from build123d import *

# Parameters (mm, degrees)
SKETCH_1_W          = 55
SKETCH_1_H          = 85
EXTRUDE_1_DEPTH     = 5
SKETCH_2_W          = 7
SKETCH_2_H          = 6.5
EXTRUDE_2_DEPTH     = 26
SKETCH_3_R          = 1.475
CUT_EXTRUDE_1_DEPTH = 103.30377559
SKETCH_4_W          = 41
SKETCH_4_H          = 15
EXTRUDE_3_DEPTH     = 7.75
SKETCH_5_W          = 24.5
SKETCH_5_H          = 49.5
EXTRUDE_4_DEPTH     = 10
SKETCH_7_R          = 2.525
CUT_EXTRUDE_2_DEPTH = 2.25
SKETCH_8_W          = 2.7
SKETCH_8_H          = 15.4
CUT_EXTRUDE_3_DEPTH = 12
SKETCH_9_W          = 1.9
SKETCH_9_H          = 14.5
CUT_EXTRUDE_4_DEPTH = 1
SKETCH_10_W         = 10
SKETCH_10_H         = 14.5
CUT_EXTRUDE_5_DEPTH = 70.787624261
FILLET_1_R          = 3
FILLET_2_R          = 7.5


with BuildPart() as part:
    # Эскиз1 → Бобышка-Вытянуть1 (new body)
    with BuildSketch(Plane(origin=(0, 0, 0), x_dir=(1, 0, 0), z_dir=(0, 1, 0))):
        with Locations((-20.25, 0)):
            Rectangle(SKETCH_1_W, SKETCH_1_H)
    extrude(amount=EXTRUDE_1_DEPTH)

    # Эскиз2 → Бобышка-Вытянуть2 (add)
    with BuildSketch(Plane(origin=(0, 5, 0), x_dir=(1, 0, 0), z_dir=(0, 1, 0))):
        with Locations((-44.25, 39.25)):
            Rectangle(SKETCH_2_W, SKETCH_2_H)
        with Locations((3.75, 39.25)):
            Rectangle(SKETCH_2_W, SKETCH_2_H)
        with Locations((3.75, -39.25)):
            Rectangle(SKETCH_2_W, SKETCH_2_H)
        with Locations((-44.25, -39.25)):
            Rectangle(SKETCH_2_W, SKETCH_2_H)
    extrude(amount=EXTRUDE_2_DEPTH)

    # Эскиз3 → Вырез-Вытянуть1 (cut, through all)
    with BuildSketch(Plane.XY.offset(42.5)):
        with Locations((-44.55, 28)):
            Circle(SKETCH_3_R)
        with Locations((-44.55, 18)):
            Circle(SKETCH_3_R)
        with Locations((4.05, 18)):
            Circle(SKETCH_3_R)
        with Locations((4.05, 28)):
            Circle(SKETCH_3_R)
    extrude(amount=-CUT_EXTRUDE_1_DEPTH, mode=Mode.SUBTRACT)

    # Эскиз4 → Бобышка-Вытянуть3 (add)
    with BuildSketch(Plane(origin=(0, 5, 0), x_dir=(1, 0, 0), z_dir=(0, 1, 0))):
        with Locations((-20.25, 35)):
            Rectangle(SKETCH_4_W, SKETCH_4_H)
        with Locations((-20.25, -35)):
            Rectangle(SKETCH_4_W, SKETCH_4_H)
    extrude(amount=EXTRUDE_3_DEPTH)

    # Эскиз5 → Бобышка-Вытянуть4 (add)
    with BuildSketch(Plane.XZ):
        with Locations((-20.25, 0)):
            Rectangle(SKETCH_5_W, SKETCH_5_H)
    extrude(amount=EXTRUDE_4_DEPTH)

    # Эскиз7 → Вырез-Вытянуть2 (cut)
    with BuildSketch(Plane.XZ.offset(10)):
        with Locations(Location((-13, 20, 0), (0, 0, 270))):
            Circle(SKETCH_7_R)
        with Locations(Location((-13, -20, 0), (0, 0, 270))):
            Circle(SKETCH_7_R)
    extrude(amount=-CUT_EXTRUDE_2_DEPTH, mode=Mode.SUBTRACT)

    # Эскиз8 → Вырез-Вытянуть3 (cut)
    with BuildSketch(Plane.XZ.offset(10)):
        with Locations((-29, 0)):
            Rectangle(SKETCH_8_W, SKETCH_8_H)
        with Locations((-25, 0)):
            Rectangle(SKETCH_8_W, SKETCH_8_H)
    extrude(amount=-CUT_EXTRUDE_3_DEPTH, mode=Mode.SUBTRACT)

    # Эскиз9 → Вырез-Вытянуть4 (cut)
    with BuildSketch(Plane.XZ.offset(-2)):
        with Locations((-29, 0)):
            Rectangle(SKETCH_9_W, SKETCH_9_H)
        with Locations((-25, 0)):
            Rectangle(SKETCH_9_W, SKETCH_9_H)
    extrude(amount=-CUT_EXTRUDE_4_DEPTH, mode=Mode.SUBTRACT)

    # Эскиз10 → Вырез-Вытянуть5 (cut, through all)
    with BuildSketch(Plane.XZ.offset(-3)):
        with Locations((-24.95, 0)):
            Rectangle(SKETCH_10_W, SKETCH_10_H)
    extrude(amount=-CUT_EXTRUDE_5_DEPTH, mode=Mode.SUBTRACT)

    # Скругление1
    fillet_1_edges = [part.edges().sort_by_distance(p)[0] for p in [
        (-32.5, -5, 24.75),
        (-32.5, -5, -24.75),
        (-8, -5, -24.75),
        (-8, -5, 24.75),
    ]]
    fillet(fillet_1_edges, radius=FILLET_1_R)

    # Скругление2
    fillet_2_edges = [part.edges().sort_by_distance(p)[0] for p in [
        (-20.25, 5, -27.5),
        (-20.25, 5, 27.5),
        (-44.25, 5, 36),
        (3.75, 5, 36),
        (3.75, 5, -36),
        (-44.25, 5, -36),
    ]]
    fillet(fillet_2_edges, radius=FILLET_2_R)


solid = part.part
Model file for the job. Use its own axes, mm. A direction names the side the tool comes from. Give positions to 0.01 mm unless a question says otherwise; leave off trailing zeros. Write each loop counter-clockwise with the first axis right and the second up, starting at its lowest first coordinate (ties: lowest second). Pieces come first, ordered by that corner, then holes. Notation, with made-up numbers: M 12,-8.5 L 16,-8.5 A20 ccw 16,12.5 Z; hole C 10,71 d10. An arc over 180 degrees is marked long. One line per item, written item: value. Start each with the question number.
Q1. Saw through at C-C, the plane z = 0. Write the cut outline in (x, y), plus the area to 3 significant figures.
Q2. Saw through at B-B, the plane y = 18. State how many separate pieces and enclosed holes the cut face has, plus the area to 3 significant figures.
Q3. Two-plate mould, pull along X, no slides. Class faces 4 (the cylindrical face through (-8.86, -5.07, 23.85)), 5 (the flat face through (-33, 0, -1)), 6 (the flat face through (-22, 3, 0)), 7 (the flat face through (-27, 3, 0)): +X half, -X half, draft (parallel to the pull), parting line (faces both ways), or undercut.
Q4. Saw through at D-D, the plane y = 10. Write the cut outline in (x, z), plus the area to 3 significant figures.
Q5. Saw through at A-A, the plane x = -44.55. Write the cut outline in (y, z) (3 decimals).
Q6. Probe probe 1 along Y at (x, z) = (4.05, 41) (3 decimals); probe 2 along Z at (x, y) = (3, 25); probe 3 along X at (y, z) = (-4.5, 0.5). List the from-to ranges inside material, lowest first. Write a range as [from, to].
Q7. 3-axis set-ups, long thin cutter, end or side, ignore diameter. For faces 1 (the flat face through (-40.75, 22, -39)), 2 (the flat face through (-29.95, 3, 0)), 3 (the flat face through (-25, 4, 7.25)): which of +Z, -Z, +X, -X, +Y, -Y reach the whole face in a straight line?
Q8. Drop flat-ended pins along their axis: pin 1 Ø2.5 at (x, z) = (-27.5, 2) entering from +Y; pin 2 Ø1 at (x, z) = (-5.5, 12.5) entering from -Y; pin 3 Ø2 at (x, y) = (-25.5, -3.5) entering from +Z; pin 4 Ø2 at (x, z) = (-28.5, 3) entering from -Y. Give the stop position or say it passes through.
Output values:
1. outline: M -47.75,0 L -32.5,0 L -32.5,-10 L -30.35,-10 L -30.35,2 L -29.95,2 L -29.95,5 L -47.75,5 Z; M -28.05,2 L -27.65,2 L -27.65,-10 L -26.35,-10 L -26.35,2 L -25.95,2 L -25.95,3 L -28.05,3 Z; M -24.05,2 L -23.65,2 L -23.65,-10 L -8,-10 L -8,0 L 7.25,0 L 7.25,5 L -19.95,5 L -19.95,3 L -24.05,3 Z
1. area: 431 mm²
2. separate pieces: 8
2. enclosed holes: 0
2. area: 105 mm²
3. face 4: +X half
3. face 5: draft
3. face 6: undercut
3. face 7: undercut
4. outline: M -47.75,-42.5 L 7.25,-42.5 L 7.25,-35.57 L 0.25,-35.57 L 0.25,-27.07 L -40.75,-27.07 L -40.75,-35.57 L -47.75,-35.57 Z; M -47.75,35.57 L -40.75,35.57 L -40.75,27.07 L 0.25,27.07 L 0.25,35.57 L 7.25,35.57 L 7.25,42.5 L -47.75,42.5 Z
4. area: 1,460 mm²
5. outline: M 0,-42.5 L 16.525,-42.5 L 16.525,-36 L 12.5,-36 A7.5 cw 5,-28.5 L 5,28.5 A7.5 cw 12.5,36 L 16.525,36 L 16.525,42.5 L 0,42.5 Z; M 19.475,-42.5 L 26.525,-42.5 L 26.525,-36 L 19.475,-36 Z; M 19.475,36 L 26.525,36 L 26.525,42.5 L 19.475,42.5 Z; M 29.475,-42.5 L 31,-42.5 L 31,-36 L 29.475,-36 Z; M 29.475,36 L 31,36 L 31,42.5 L 29.475,42.5 Z
6. probe 1: y = [0, 16.525], [19.475, 26.525], [29.475, 31]
6. probe 2: z = [-42.5, -36], [36, 42.5]
6. probe 3: x = [-32.5, -30.35], [-27.65, -26.35], [-23.65, -8]
7. face 1: +Z, -Z, +Y
7. face 2: +Y, -Y
7. face 3: +Y
8. pin 1: stops at y = 3
8. pin 2: stops at y = 0
8. pin 3: stops at z = 24.75
8. pin 4: stops at y = -10
